CAD build for the part. Positions are in the model's coordinates, mm. Give positions to 0.01 mm unless a question says otherwise; leave off trailing zeros. Loops run counter-clockwise (first coordinate to the right, second up) from the corner with the lowest first, then second, coordinate; pieces in that order, holes last. Notation, with made-up numbers: (64.25, -37) -> (116.25, -37) arc R14 ccw to (116.25, -12) -> close; hole circle Ø7 at (-39.75, -28.75). An arc over 180 degrees is marked (long way). Use one line per item in the form item = value.
```python
from build123d import *

# Parameters (mm, degrees)
F0_W     = 20
F0_H     = 20
F1_DEPTH = 1
F2_W     = 0.05
F2_H     = 10
F3_DEPTH = 25
F5_D     = 2.5


with BuildPart() as f1:
    # F0 (on Top) → F1 (new body)
    with BuildSketch(Plane.XY):
        Rectangle(F0_W, F0_H)
    extrude(amount=F1_DEPTH)

    # F2 (on face) → F3 (cut)
    with BuildSketch(Plane.XY.offset(1)):
        Rectangle(F2_W, F2_H)
    extrude(amount=-F3_DEPTH, mode=Mode.SUBTRACT)

    # F5 (through all)
    with Locations(Plane.XY.offset(1)):
        with Locations((-7, -7), (7, -7), (7, 7), (-7, 7)):
            Hole(F5_D / 2)


solid = f1.part
```
1. Cut at A-A, the plane x = -7. Write the cut outline in (y, z), then the cut area to 3 significant figures.
Result sheet:
outline = (-10, 0) -> (-8.25, 0) -> (-8.25, 1) -> (-10, 1) -> close; (-5.75, 0) -> (5.75, 0) -> (5.75, 1) -> (-5.75, 1) -> close; (8.25, 0) -> (10, 0) -> (10, 1) -> (8.25, 1) -> close
area = 15.0 mm^2
2. Mould opens along X. For faces 1 (the flat face through (10, -0.1, 0.5)), 2 (the flat face through (-10, -0.1, 0.5)), 3 (the cylindrical face through (-6.01, 6.24, 0.49)) say: pulls with the +X half, pulls with the -X half, needs draft (parallel to the pull), parting line crosses it, or undercut.
Result sheet:
face_1 = pulls with the +X half
face_2 = pulls with the -X half
face_3 = undercut
3. Cut at B-B, the plane z = 0.7. Write the cut outline in (x, y) (3 decimals), then the cut area to 3 significant figures.
Result sheet:
outline = (-10, -10) -> (10, -10) -> (10, 10) -> (-10, 10) -> close; hole circle Ø2.5 at (-7, -7); hole circle Ø2.5 at (-7, 7); hole (-0.025, -5) -> (0.025, -5) -> (0.025, 5) -> (-0.025, 5) -> close; hole circle Ø2.5 at (7, -7); hole circle Ø2.5 at (7, 7)
area = 380 mm^2
4. Drill centre lines: line 1 (Y direction, x = 7.25, z = 0.5); line 2 (Y direction, x = 8, z = 0.55). Where is each one in solid material? Low to high.
Result sheet:
line_1 = -10 to -8.22, -5.78 to 5.78, 8.22 to 10
line_2 = -10 to -7.75, -6.25 to 6.25, 7.75 to 10
